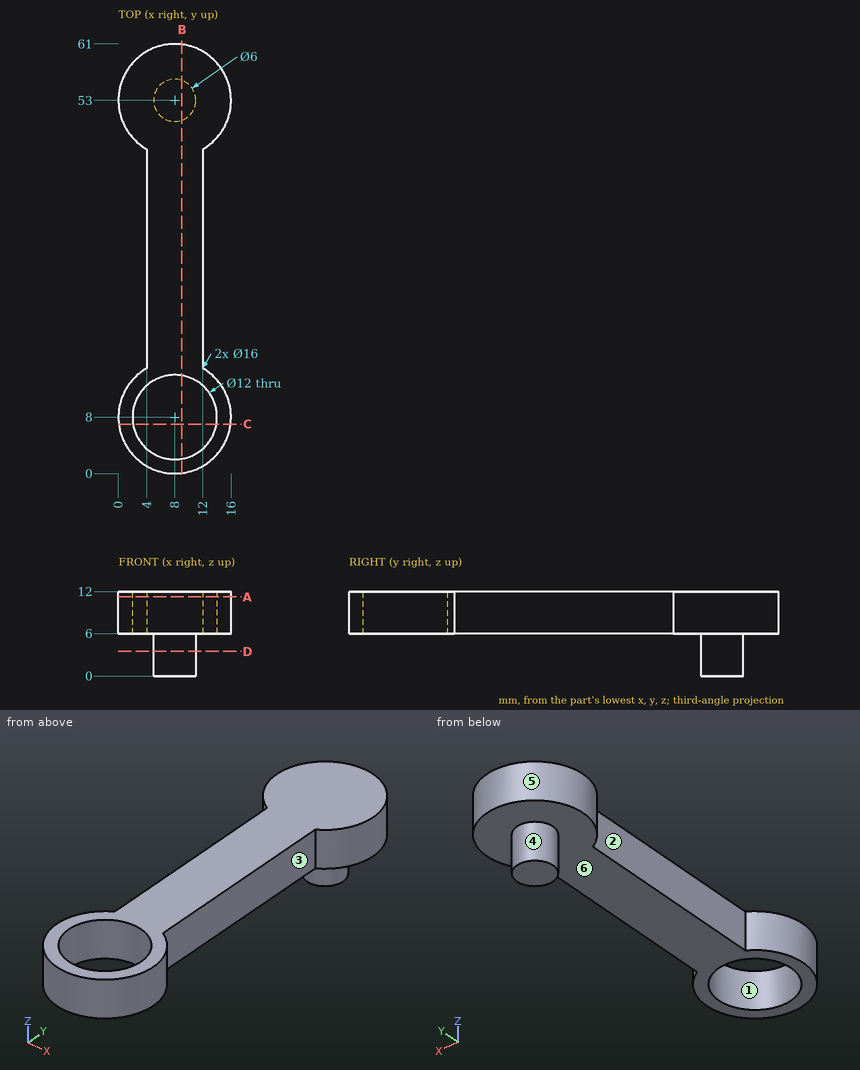
Geometry check sheet. Reference: drawing and pictorial views, mm from the part's lowest x, y, z. A direction names the side the tool comes from. Round coordinates to 2 decimals unless told otherwise and drop trailing zeros. Write each loop counter-clockwise with the first axis right and the second up, starting at its lowest first coordinate (ties: lowest second). Pieces come first, ordered by that corner, then holes. Notation, with made-up numbers: (14, 74) -> (38, 74) arc R28 cw to (38, 102) -> close; hole circle Ø9 at (75, 48). An arc over 180 degrees is marked (long way). Answer as CSV lines item,"result". Start each with the question number.
1) Section check B-B on x = 9. Enter the section's corners in (y, z).
2) Section check A-A on z = 11.25. Enter the section's corners in (x, y), and give its area (3 significant figures).
3) Go/stop test with flat-tipped pins: P1, Ø4, axis at x = 12, y = 38.5, coming from the -Z side; P2, Ø4, axis at y = 28, z = 5.5, coming from the +X side; P3, Ø2, axis at y = 21, z = 4.5, coming from the -X side; P4, Ø4, axis at x = 2.5, z = 6.5, coming from the +Y side. Record where each tip stops, or that it passes through.
4) Release check for a two-part mould opening along Y. For the marked faces 4, 5 and 6 record: pulls with the +Y half, pulls with the -Y half, needs draft (parallel to the pull), parting line crosses it, or undercut.
5) Material ranges on line 1 (Y direction, x = 2.75, z = 10.5); line 2 (Y direction, x = 1.5, z = 9.25); line 3 (Y direction, x = 9.5, z = 11.75), recorded low to high. Write a range as from..to.
6) Section check D-D on z = 3.5. Enter the section's corners in (x, y), and give its area (3 significant figures).
7) Tool access check on the marked faces 1, 2 and 3. Record the directions out of +Z, -Z, +X, -X, +Y, -Y that give a thin tool (end or side, any length) a straight path to the whole face; none if there is none.
8) Section check C-C on y = 7. Enter the section's corners in (x, z).
Found:
1,outline,"(0.06, 6) -> (2.08, 6) -> (2.08, 12) -> (0.06, 12) -> close; (13.92, 6) -> (50.17, 6) -> (50.17, 0) -> (55.83, 0) -> (55.83, 6) -> (60.94, 6) -> (60.94, 12) -> (13.92, 12) -> close"
2,outline,"(4, 14.93) arc R8 ccw (long way) to (12, 14.93) -> (12, 46.07) arc R8 ccw (long way) to (4, 46.07) -> close; hole circle Ø12 at (8, 8)"
2,area,"527 mm^2"
3,P1,"stops at z = 6"
3,P2,"stops at x = 12"
3,P3,"passes through"
3,P4,"stops at y = 60.19"
4,face 4,"parting line crosses it"
4,face 5,"undercut"
4,face 6,"needs draft"
5,line 1,"y = 1.96..5.1, 10.9..14.04, 46.96..59.04"
5,line 2,"y = 3.34..12.66, 48.34..57.66"
5,line 3,"y = 0.14..2.19, 13.81..60.86"
6,outline,"circle Ø6 at (8, 53)"
6,area,"28.3 mm^2"
7,face 1,"+Z, -Z"
7,face 2,"+Z, -Z, -X"
7,face 3,"+Z, -Z, +X"
8,outline,"(0.06, 6) -> (2.08, 6) -> (2.08, 12) -> (0.06, 12) -> close; (13.92, 6) -> (15.94, 6) -> (15.94, 12) -> (13.92, 12) -> close"
